from build123d import *

# Parameters (mm, degrees)
SKIZZE1_W                       = 450
SKIZZE1_H                       = 310
AUFSATZ_LINEAR_AUSTRAGEN1_DEPTH = 5
SKIZZE2_W                       = 10
SKIZZE2_H                       = 10
SKIZZE2_W_2                     = 25
SCHNITT_LINEAR_AUSTRAGEN1_DEPTH = 547.465918425
SKIZZE3_W                       = 5
SKIZZE3_H                       = 100
SCHNITT_LINEAR_AUSTRAGEN2_DEPTH = 547.465918425
SKIZZE4_R                       = 1.5
SCHNITT_LINEAR_AUSTRAGEN3_DEPTH = 547.465918425
SKIZZE5_W                       = 2
SKIZZE5_H                       = 290
SKIZZE5_W_2                     = 60
SKIZZE5_H_2                     = 2
SKIZZE5_W_3                     = 220
SKIZZE5_W_4                     = 100
SCHNITT_LINEAR_AUSTRAGEN4_DEPTH = 547.465918425


with BuildPart() as part:
    # Skizze1 → Aufsatz-Linear austragen1 (new body)
    with BuildSketch(Plane(origin=(0, 0, 0), x_dir=(1, 0, 0), z_dir=(0, 1, 0))):
        with Locations((225, -155)):
            Rectangle(SKIZZE1_W, SKIZZE1_H)
    extrude(amount=AUFSATZ_LINEAR_AUSTRAGEN1_DEPTH)

    # Skizze2 → Schnitt-Linear austragen1 (cut, through all)
    with BuildSketch(Plane(origin=(0, 5, 0), x_dir=(1, 0, 0), z_dir=(0, 1, 0))):
        with Locations((5, -5)):
            Rectangle(SKIZZE2_W, SKIZZE2_H)
        with Locations((445, -305)):
            Rectangle(SKIZZE2_W, SKIZZE2_H)
        with Locations((445, -5)):
            Rectangle(SKIZZE2_W, SKIZZE2_H)
        with Locations((5, -305)):
            Rectangle(SKIZZE2_W, SKIZZE2_H)
        with Locations((82.5, -5)):
            Rectangle(SKIZZE2_W_2, SKIZZE2_H)
        with Locations((327.5, -5)):
            Rectangle(SKIZZE2_W_2, SKIZZE2_H)
        with Locations((327.5, -305)):
            Rectangle(SKIZZE2_W_2, SKIZZE2_H)
        with Locations((82.5, -305)):
            Rectangle(SKIZZE2_W_2, SKIZZE2_H)
    extrude(amount=-SCHNITT_LINEAR_AUSTRAGEN1_DEPTH, mode=Mode.SUBTRACT)

    # Skizze3 → Schnitt-Linear austragen2 (cut, through all)
    with BuildSketch(Plane(origin=(0, 5, 0), x_dir=(1, 0, 0), z_dir=(0, 1, 0))):
        with Locations((112.5, -155)):
            Rectangle(SKIZZE3_W, SKIZZE3_H)
        with Locations((297.5, -155)):
            Rectangle(SKIZZE3_W, SKIZZE3_H)
    extrude(amount=-SCHNITT_LINEAR_AUSTRAGEN2_DEPTH, mode=Mode.SUBTRACT)

    # Skizze4 → Schnitt-Linear austragen3 (cut, through all)
    with BuildSketch(Plane(origin=(0, 5, 0), x_dir=(1, 0, 0), z_dir=(0, 1, 0))):
        with Locations(Location((40, -10, 0), (0, 0, 270))):
            Circle(SKIZZE4_R)
        with Locations(Location((205, -10, 0), (0, 0, 270))):
            Circle(SKIZZE4_R)
        with Locations(Location((390, -10, 0), (0, 0, 270))):
            Circle(SKIZZE4_R)
        with Locations(Location((40, -300, 0), (0, 0, 270))):
            Circle(SKIZZE4_R)
        with Locations(Location((205, -300, 0), (0, 0, 270))):
            Circle(SKIZZE4_R)
        with Locations(Location((390, -300, 0), (0, 0, 270))):
            Circle(SKIZZE4_R)
    extrude(amount=-SCHNITT_LINEAR_AUSTRAGEN3_DEPTH, mode=Mode.SUBTRACT)

    # Skizze5 → Schnitt-Linear austragen4 (cut, through all)
    with BuildSketch(Plane(origin=(0, 5, 0), x_dir=(1, 0, 0), z_dir=(0, 1, 0))):
        with Locations((0, -155)):
            Rectangle(SKIZZE5_W, SKIZZE5_H)
        with Locations((40, 0)):
            Rectangle(SKIZZE5_W_2, SKIZZE5_H_2)
        with Locations((205, 0)):
            Rectangle(SKIZZE5_W_3, SKIZZE5_H_2)
        with Locations((390, 0)):
            Rectangle(SKIZZE5_W_4, SKIZZE5_H_2)
        with Locations((450, -155)):
            Rectangle(SKIZZE5_W, SKIZZE5_H)
        with Locations((390, -310)):
            Rectangle(SKIZZE5_W_4, SKIZZE5_H_2)
        with Locations((205, -310)):
            Rectangle(SKIZZE5_W_3, SKIZZE5_H_2)
        with Locations((40, -310)):
            Rectangle(SKIZZE5_W_2, SKIZZE5_H_2)
    extrude(amount=-SCHNITT_LINEAR_AUSTRAGEN4_DEPTH, mode=Mode.SUBTRACT)


solid = part.part
CAD build for the part. Positions are in the model's coordinates, mm. Coordinates: 2 decimals unless noted, no trailing zeros. Order: outer loops, then holes, each group sorted by start corner. A loop starts at its lowest first (then second) coordinate and runs counter-clockwise, first axis right, second up.
Item 1: Drill centre lines: L1, parallel to Z at x = 390, y = 4; L2, parallel to X at y = 3.95, z = 198. Where is each one in solid material? Low to high.
Check sheet entries:
L1: z = 1 to 8.5, 11.5 to 298.5, 301.5 to 309
L2: x = 1 to 110, 115 to 295, 300 to 449
Item 2: Band-saw the part on A-A on z = 167. List the corners of the cut face in (x, y), plus the area to 3 significant figures.
Check sheet entries:
outline: (1, 0) - (110, 0) - (110, 5) - (1, 5) - close; (115, 0) - (295, 0) - (295, 5) - (115, 5) - close; (300, 0) - (449, 0) - (449, 5) - (300, 5) - close
area: 2,190 mm2
Item 3: Band-saw the part on B-B on y = 1.4. Give the number of separate pieces and of enclosed holes in the cut face, plus the area to 3 significant figures.
Check sheet entries:
separate pieces: 1
enclosed holes: 8
area: 136,000 mm2
Item 4: Pin check, flat tips, straight feed: pin 1 Ø2.5 at (y, z) = (1.5, 6) entering from +X; pin 2 Ø1.8 at (x, z) = (40, 300) entering from +Y; pin 3 Ø1 at (x, z) = (105.5, 198.5) entering from -Y; pin 4 Ø2.5 at (x, y) = (442.5, 2.5) entering from -Z. Stop position of each tip, or through.
Check sheet entries:
pin 1: stops at x = 440
pin 2: passes through
pin 3: stops at y = 0
pin 4: stops at z = 10
